Part model, mm, in its own coordinate system. Face numbers are marked on the shaded views. Give positions to 0.01 mm unless a question says otherwise; leave off trailing zeros. Write each loop counter-clockwise with the first axis right and the second up, starting at its lowest first coordinate (ties: lowest second). Pieces come first, ordered by that corner, then holes. Notation, with made-up numbers: M -17.5,-38.5 L 34.5,-38.5 A33 ccw 34.5,-9.5 Z; hole C 89.25,36 d3. An arc over 180 degrees is marked long. Use CSV: the item, a comma, the result in double quotes. Start each with the question number.
1. Band-saw the part on B-B, the plane x = 0. List the corners of the cut face in (y, z).
2. Band-saw the part on D-D, the plane z = 7. List the corners of the cut face in (x, y), then the cut area to 3 significant figures.
3. Mould opens along Z. For the marked faces 1, 2 and 3 say: pulls with the +Z half, pulls with the -Z half, needs draft (parallel to the pull), parting line crosses it, or undercut.
4. Drop flat-ended pins along their axis: pin 1 Ø2 at (x, z) = (-9.5, -7.5) entering from -Y; pin 2 Ø4 at (x, y) = (-3.5, 7) entering from +Z; pin 3 Ø3 at (x, y) = (6.5, 9.5) entering from -Z. Give the stop position or say it passes through.
5. Drill centre lines: line 1 along X through (y, z) = (4, 0); line 2 along X through (y, z) = (17.5, -2); line 3 along Y through (x, z) = (-4.5, -6.5). Where is each one in solid material? Low to high. Write a range as from..to.
6. Band-saw the part on A-A, the plane z = 0. List the corners of the cut face in (x, y), then the cut area to 3 significant figures.
7. Band-saw the part on C-C, the plane y = 5.5. List the corners of the cut face in (x, z), then the cut area to 3 significant figures.
from build123d import *

# Parameters (mm, degrees)
SKETCH2_R           = 16
BOSS_EXTRUDE1_DEPTH = 20
CUT_EXTRUDE1_START  = -2
SKETCH3_R           = 15
CUT_EXTRUDE1_DEPTH  = 29.199337741
SKETCH4_R           = 3
BOSS_EXTRUDE2_DEPTH = 1


with BuildPart() as part:
    # Sketch2 → Boss-Extrude1 (new body)
    with BuildSketch(Plane(origin=(0, 0, 0), x_dir=(1, 0, 0), z_dir=(0, 1, 0))):
        with Locations(Location((0, 0, 0), (0, 0, 270))):
            Circle(SKETCH2_R)
    extrude(amount=BOSS_EXTRUDE1_DEPTH)

    # Sketch3 → Cut-Extrude1 (cut, through all)
    with BuildSketch(Plane(origin=(0, 20, 0), x_dir=(1, 0, 0), z_dir=(0, 1, 0)).offset(CUT_EXTRUDE1_START)):
        with Locations(Location((0, 0, 0), (0, 0, 270))):
            Circle(SKETCH3_R)
    extrude(amount=-CUT_EXTRUDE1_DEPTH, mode=Mode.SUBTRACT)

    # Sketch4 → Boss-Extrude2 (add)
    with BuildSketch(Plane(origin=(0, 18, 0), x_dir=(-1, 0, 0), z_dir=(0, -1, 0))):
        with Locations(Location((0, 0, 0), (0, 0, 270))):
            Circle(SKETCH4_R)
    extrude(amount=BOSS_EXTRUDE2_DEPTH)


solid = part.part
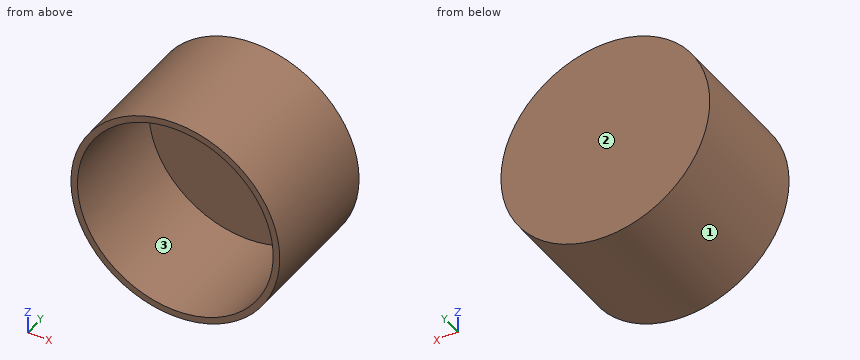
Output:
1,outline,"M 0,-16 L 20,-16 L 20,16 L 0,16 L 0,15 L 18,15 L 18,3 L 17,3 L 17,-3 L 18,-3 L 18,-15 L 0,-15 Z"
2,outline,"M -14.39,0 L -13.27,0 L -13.27,18 L 13.27,18 L 13.27,0 L 14.39,0 L 14.39,20 L -14.39,20 Z"
2,area,"97.9 mm²"
3,face 1,"parting line crosses it"
3,face 2,"needs draft"
3,face 3,"undercut"
4,pin 1,"stops at y = 18"
4,pin 2,"stops at z = 15.93"
4,pin 3,"stops at z = -15.2"
5,line 1,"x = -16..-15, 15..16"
5,line 2,"x = -15.87..-14.87, -2.24..2.24, 14.87..15.87"
5,line 3,"y = 18..20"
6,outline,"M -16,0 L -15,0 L -15,18 L -3,18 L -3,17 L 3,17 L 3,18 L 15,18 L 15,0 L 16,0 L 16,20 L -16,20 Z"
6,area,"106 mm²"
7,outline,"C 0,0 d32; hole C 0,0 d30"
7,area,"97.4 mm²"
